```python
from build123d import *

# Parameters (mm, degrees)
F1_DEPTH = 10
F2_DEPTH = 25


with BuildPart() as f1:
    # F0 (on Top) → F1 (new body)
    with BuildSketch(Plane.XY):
        with BuildLine():
            Line((2.8350751381, 17.25), (2.8350751381, 15.84981649))
            ThreePointArc((2.8350751381, 15.84981649), (5.8670915268, 18.4319851995), (7, 22.25))
            ThreePointArc((7, 22.25), (-3.8180148005, 28.1170915268), (-2.8350751381, 15.84981649))
            Line((-2.8350751381, 15.84981649), (-2.8350751381, 17.25))
            Line((-2.8350751381, 17.25), (0, 17.25))
            Line((0, 17.25), (2.8350751381, 17.25))
        make_face()
        with BuildLine():
            ThreePointArc((5, 22.25), (3.5355339059, 18.7144660941), (0, 17.25))
            ThreePointArc((0, 17.25), (-3.5355339059, 25.7855339059), (5, 22.25))
        make_face(mode=Mode.SUBTRACT)
        with BuildLine():
            ThreePointArc((-2.8350751381, 15.84981649), (0, 15.25), (2.8350751381, 15.84981649))
            Line((2.8350751381, 15.84981649), (2.8350751381, 17.25))
            Line((2.8350751381, 17.25), (0, 17.25))
            Line((0, 17.25), (-2.8350751381, 17.25))
            Line((-2.8350751381, 17.25), (-2.8350751381, 15.84981649))
        make_face()
        with BuildLine():
            ThreePointArc((-2.8350751381, 9.8501192359), (0, 10.25), (2.8350751381, 9.8501192359))
            Line((2.8350751381, 9.8501192359), (2.8350751381, 15.84981649))
            ThreePointArc((2.8350751381, 15.84981649), (0, 15.25), (-2.8350751381, 15.84981649))
            Line((-2.8350751381, 15.84981649), (-2.8350751381, 9.8501192359))
        make_face()
        with BuildLine():
            Line((-2.8350751381, 8.25), (0, 8.25))
            Line((0, 8.25), (2.8350751381, 8.25))
            Line((2.8350751381, 8.25), (2.8350751381, 9.8501192359))
            ThreePointArc((2.8350751381, 9.8501192359), (0, 10.25), (-2.8350751381, 9.8501192359))
            Line((-2.8350751381, 9.8501192359), (-2.8350751381, 8.25))
        make_face()
        with BuildLine():
            Line((2.8350751381, 8.25), (0, 8.25))
            Line((0, 8.25), (-2.8350751381, 8.25))
            Line((-2.8350751381, 8.25), (-2.8350751381, 9.8501192359))
            ThreePointArc((-2.8350751381, 9.8501192359), (-6.16453485, -8.1890787078), (10.25, 0))
            ThreePointArc((10.25, 0), (8.1890787078, 6.16453485), (2.8350751381, 9.8501192359))
            Line((2.8350751381, 9.8501192359), (2.8350751381, 8.25))
        make_face()
        with BuildLine():
            ThreePointArc((0, 8.25), (5.8336309448, 5.8336309448), (8.25, 0))
            ThreePointArc((8.25, 0), (-5.8336309448, -5.8336309448), (0, 8.25))
        make_face(mode=Mode.SUBTRACT)
    extrude(amount=F1_DEPTH)

    # F0 (on Top) → F2 (join)
    with BuildSketch(Plane.XY):
        with BuildLine():
            Line((2.8350751381, 17.25), (2.8350751381, 15.84981649))
            ThreePointArc((2.8350751381, 15.84981649), (5.8670915268, 18.4319851995), (7, 22.25))
            ThreePointArc((7, 22.25), (-3.8180148005, 28.1170915268), (-2.8350751381, 15.84981649))
            Line((-2.8350751381, 15.84981649), (-2.8350751381, 17.25))
            Line((-2.8350751381, 17.25), (0, 17.25))
            Line((0, 17.25), (2.8350751381, 17.25))
        make_face()
        with BuildLine():
            ThreePointArc((5, 22.25), (3.5355339059, 18.7144660941), (0, 17.25))
            ThreePointArc((0, 17.25), (-3.5355339059, 25.7855339059), (5, 22.25))
        make_face(mode=Mode.SUBTRACT)
        with BuildLine():
            ThreePointArc((-2.8350751381, 15.84981649), (0, 15.25), (2.8350751381, 15.84981649))
            Line((2.8350751381, 15.84981649), (2.8350751381, 17.25))
            Line((2.8350751381, 17.25), (0, 17.25))
            Line((0, 17.25), (-2.8350751381, 17.25))
            Line((-2.8350751381, 17.25), (-2.8350751381, 15.84981649))
        make_face()
    extrude(amount=F2_DEPTH)


solid = f1.part
```
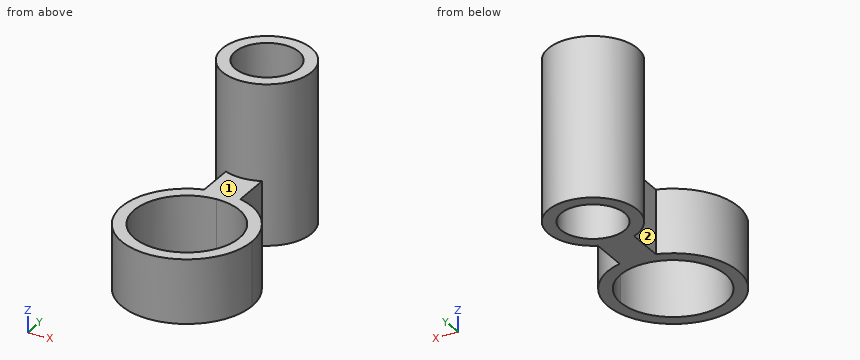
The listing builds one solid part. Answer for the finished solid, in the listing's coordinates (mm). Face numbers are marked on the shaded views. Coordinates: 2 decimals unless noted, no trailing zeros. Loops run counter-clockwise (first coordinate to the right, second up) from the corner with the lowest first, then second, coordinate; pieces in that order, holes last. Notation, with made-up numbers: M 83.5,-7 L 89.5,-7 A10 cw 89.5,5 Z; hole C 23,70 d10. An arc over 180 degrees is marked long. Answer as a JSON object with one key per item and string values. Group by question number.
Item 1: Each of these flat-tipped pins is pushed along its axis until it touches: P1, Ø8, axis at x = 0, y = 22.25, coming from the -Z side; P2, Ø5, axis at x = -7.5, z = 11.5, coming from the +Y side; P3, Ø1.8, axis at y = 12.5, z = 7.5, coming from the -X side; P4, Ø6, axis at x = -2, y = 8, coming from the +Z side. Where does it stop, or does it pass through?
Item 2: Determine the mould class of the marked faces 1 and 2 for opening direction Y: +Y half, -Y half, draft (parallel to the pull), parting line (faces both ways), or undercut.
Item 3: Section A-A (y = 22.25) is taken. Write down the section's boundary in (x, z).
Item 4: Consider L1, parallel to X at y = 22.25, z = 19.75; L2, parallel to X at y = 0, z = 5.25; L3, parallel to Y at x = -0.75, z = 4. Determine where each line is inside the solid, lowest interval first.
Item 5: Section C-C (x = 3.75) is taken. Write down the section's boundary in (y, z), and give its area (3 significant figures).
Item 6: Section D-D (z = 12.5) is taken. Write down the section's boundary in (x, y).
Item 7: Section B-B (z = 8.25) is taken. Write down the section's boundary in (x, y).
Solved:
{
 "1": {"P1": "passes through", "P2": "stops at y = 27.15", "P3": "stops at x = -2.84", "P4": "stops at z = 10"},
 "2": {"face 1": "draft", "face 2": "undercut"},
 "3": {"outline": "M -7,0 L -5,0 L -5,25 L -7,25 Z; M 5,0 L 7,0 L 7,25 L 5,25 Z"},
 "4": {"L1": "x = -7 to -5, 5 to 7", "L2": "x = -10.25 to -8.25, 8.25 to 10.25", "L3": "y = -10.22 to -8.22, 8.22 to 17.31, 27.19 to 29.21"},
 "5": {"outline": "M -9.54,0 L -7.35,0 L -7.35,10 L -9.54,10 Z; M 7.35,0 L 9.54,0 L 9.54,10 L 7.35,10 Z; M 16.34,0 L 18.94,0 L 18.94,25 L 16.34,25 Z; M 25.56,0 L 28.16,0 L 28.16,25 L 25.56,25 Z", "area": "174 mm2"},
 "6": {"outline": "C 0,22.25 d14; hole C 0,22.25 d10"},
 "7": {"outline": "M -2.84,9.85 A10.25 ccw long 2.84,9.85 L 2.84,15.85 A7 ccw long -2.84,15.85 Z; hole C 0,0 d16.5; hole C 0,22.25 d10"}
}
